```python
from build123d import *

# Parameters (mm, degrees)
F1_DEPTH     = 15
F3_DEPTH     = 6
F5_DEPTH     = 18
F6_R         = 10
F9_DEPTH     = 6
F10_DEPTH    = 6
F11_R        = 2
F13_DEPTH    = 6
F15_R        = 10
F19_DEPTH    = 45.001
F21_DEPTH    = 40.001
F23_DEPTH    = 6
F24_T1_DEPTH = 6


# Not quite as in the source:
# - a fillet or chamfer that OpenCascade refuses, or shapes differently, is made with other operations: its cross-section is extruded or revolved along the edge and cut away or added


with BuildPart() as f1:
    # F0 (on Front) → F1 (new body, symmetric)
    with BuildSketch(Plane.XZ):
        Polygon((9, -15), (9, 15), (3, 15), (3, 25), (-3, 25), (-3, 15), (-9, 15), (-9, -15), (-9, -25), (-3, -25), (-3, -15), (3, -15), (3, -25), (9, -25), align=None)
    extrude(amount=F1_DEPTH, both=True)

    # F2 (on face) → F3 (cut)
    with BuildSketch(Plane(origin=(-3, 0, 0), x_dir=(0, -1, 0), z_dir=(-1, 0, 0))):
        with BuildLine():
            ThreePointArc((0, 22.62), (-2.62, 20), (0, 17.38))
            Line((0, 17.38), (0, 22.62))
        make_face()
        with BuildLine():
            Line((0, 22.62), (0, 17.38))
            ThreePointArc((0, 17.38), (1.8526197667, 18.1473802333), (2.62, 20))
            ThreePointArc((2.62, 20), (1.8526197667, 21.8526197667), (0, 22.62))
        make_face()
    extrude(amount=-F3_DEPTH, mode=Mode.SUBTRACT)

    # F4 (on face) → F5 (cut)
    with BuildSketch(Plane(origin=(-9, 0, 0), x_dir=(0, -1, 0), z_dir=(-1, 0, 0))):
        with BuildLine():
            ThreePointArc((0, -22.62), (1.8526197667, -21.8526197667), (2.62, -20))
            ThreePointArc((2.62, -20), (-1.8526197667, -18.1473802333), (0, -22.62))
        make_face()
    extrude(amount=-F5_DEPTH, mode=Mode.SUBTRACT)

    # F6
    f6_edges = [f1.edges().sort_by_distance(p)[0] for p in [
        (0, 15, 25),
        (0, -15, 25),
        (6, -15, -25),
        (-6, -15, -25),
    ]]
    fillet(f6_edges, radius=F6_R)

    # F8 (on face) → F9 (cut)
    with BuildSketch(Plane(origin=(-9, 0, 0), x_dir=(0, -1, 0), z_dir=(-1, 0, 0))):
        with BuildLine():
            ThreePointArc((-7, 13.5872004348), (-5.1915204429, 7.8514360713), (-0.4202014333, 4.190274227))
            Line((-0.4202014333, 4.190274227), (15, -1.4222201011))
            Line((15, -1.4222201011), (15, 15))
            Line((15, 15), (-7, 15))
            Line((-7, 15), (-7, 13.5872004348))
        make_face()
    extrude(amount=-F9_DEPTH, mode=Mode.SUBTRACT)

    # F7 (on face) → F10 (cut)
    with BuildSketch(Plane.YZ.offset(9)):
        with BuildLine():
            Line((7, 15), (-15, 15))
            Line((-15, 15), (-15, -1.42222))
            Line((-15, -1.42222), (0.4202014333, 4.1902743281))
            ThreePointArc((0.4202014333, 4.1902743281), (5.1915204429, 7.8514361724), (7, 13.587200536))
            Line((7, 13.587200536), (7, 15))
        make_face()
    extrude(amount=-F10_DEPTH, mode=Mode.SUBTRACT)

    # F11
    f11_edges = [f1.edges().sort_by_distance(p)[0] for p in [
        (9, 15, -5),
        (-9, 15, -5),
    ]]
    fillet(f11_edges, radius=F11_R)

    # F12 (on face) → F13 (cut)
    with BuildSketch(Plane(origin=(-3, 0, 0), x_dir=(0, -1, 0), z_dir=(-1, 0, 0))):
        with BuildLine():
            Line((5, 25), (0, 25))
            ThreePointArc((0, 25), (3.5355339059, 23.5355339059), (5, 20))
            Line((5, 20), (5, 2.2174822415))
            Line((5, 2.2174822415), (15, -1.4222201011))
            Line((15, -1.4222201011), (15, 15))
            ThreePointArc((15, 15), (12.0710678119, 22.0710678119), (5, 25))
        make_face()
    extrude(amount=-F13_DEPTH, mode=Mode.SUBTRACT)

    # F15
    f15_edges = [f1.edges().sort_by_distance(p)[0] for p in [
        (0, -15, -15),
    ]]
    fillet(f15_edges, radius=F15_R)

    # F18 (on face) → F19 (cut, through all)
    with BuildSketch(Plane.XY.offset(20)):
        with BuildLine():
            ThreePointArc((2, -10), (1.4142135624, -8.5857864376), (0, -8))
            Line((0, -8), (0, -12))
            ThreePointArc((0, -12), (1.4142135624, -11.4142135624), (2, -10))
        make_face()
        with BuildLine():
            Line((0, -12), (0, -8))
            ThreePointArc((0, -8), (-2, -10), (0, -12))
        make_face()
    extrude(amount=-F19_DEPTH, mode=Mode.SUBTRACT)

    # F20 (on face) → F21 (cut, through all)
    with BuildSketch(Plane(origin=(0, 0, -15), x_dir=(1, 0, 0), z_dir=(0, 0, -1))):
        with BuildLine():
            ThreePointArc((0, -9), (-2, -11), (0, -13))
            Line((0, -13), (0, -11))
            Line((0, -11), (0, -9))
        make_face()
        with BuildLine():
            Line((0, -11), (0, -13))
            ThreePointArc((0, -13), (1.4142135624, -12.4142135624), (2, -11))
            ThreePointArc((2, -11), (1.4142135624, -9.5857864376), (0, -9))
            Line((0, -9), (0, -11))
        make_face()
    extrude(amount=-F21_DEPTH, mode=Mode.SUBTRACT)

    # F22 (on face) → F23 (cut)
    with BuildSketch(Plane.YZ.offset(3)):
        with BuildLine():
            ThreePointArc((0, 15), (-3.5355339059, 16.4644660941), (-5, 20))
            Line((-5, 20), (-5, 2.2174822415))
            Line((-5.0000000325, 2.2174823308), (0, 4.037333514))
            Line((0, 4.037333514), (0, 15))
        make_face()
    extrude(amount=-F23_DEPTH, mode=Mode.SUBTRACT)

    # F24: fillet of radius 5 on 2 edges, made by hand

    # F24_s2 → F24_t1 (join)
    with BuildSketch(Plane.YZ.offset(-3)):
        with BuildLine():
            ThreePointArc((-2.5, 15.6698729811), (-0.6698729811, 13.8397459622), (0, 11.3397459622))
            Line((0, 11.3397459622), (0, 15))
            ThreePointArc((0, 15), (-1.2940952255, 15.1703708686), (-2.5, 15.6698729811))
        make_face()
        with BuildLine():
            ThreePointArc((-3.2898992834, 2.8399081011), (-0.9042397786, 4.6704890233), (0, 7.538371205))
            Line((0, 7.538371205), (0, 4.037333514))
            Line((0, 4.037333514), (-3.2898992834, 2.8399081011))
        make_face()
    extrude(amount=F24_T1_DEPTH)


solid = f1.part
```
CAD build for the part. Positions are in the model's coordinates, mm. A direction names the side the tool comes from. Round coordinates to 2 decimals unless told otherwise and drop trailing zeros. Loops run counter-clockwise (first coordinate to the right, second up) from the corner with the lowest first, then second, coordinate; pieces in that order, holes last. Notation, with made-up numbers: M -5.75,-15 L 32.25,-15 A19 ccw 32.25,-5 Z; hole C 73,28.25 d1. An arc over 180 degrees is marked long. Use a Markdown table: item, result. Add a question column.
(1) Which spindle directions (+Z, -Z, +X, -X, +Y, -Y) get a long thin tool onto all of the face, cutting with end or side? Do faces 1 (the face through (0, 0, 9)), 2 (the face through (6, 7, 14)), 3 (the face through (6, 11, 15)), 4 (the face through (0, 5, -15)). Say none if no direction does.
(2) Pull direction X, two halves, no side cores. Call faces 5 (the face through (8.4, 14.43, -4.72)), 6 (the face through (0, -13, -11)), 7 (the face through (-8.4, 14.43, -5.28)): +X half, -X half, draft (parallel to the pull), parting line (faces both ways), or undercut.
(3) Drill centre lines: line 1 (Y direction, x = -4.2, z = -20); line 2 (X direction, y = 10, z = -17); line 3 (Z direction, x = 5.25, y = -1.5). Where is each one in solid material? Low to high.
(4) Cut at A-A (x = 4). Give the cut face in (y, z).
(5) Cut at C-C (z = -10). Give the cut face in (x, y), and give its area (3 significant figures).
(6) Cut at D-D (x = -0.75). Give the cut face in (y, z).
(7) Cut at B-B (z = -18). Give the cut face in (x, y).
(8) Flat gauge pins, fed straight in: pin 1 (10 mm diameter, centred on y = 1.5, z = 12.5, fed in from -X); pin 2 (3 mm diameter, centred on x = -5, y = 9, fed in from +Z); pin 3 (1.8 mm diameter, centred on x = 1.5, y = 2, fed in from -Z). Where does each tip first touch, or does it go through?
Geometry says:
| question | item | result |
|---|---|---|
| 1 | face 1 | +X, -X, -Y |
| 1 | face 2 | +Z, +X, -Y |
| 1 | face 3 | +Z, +X, +Y, -Y |
| 1 | face 4 | -Z, +Y, -Y |
| 2 | face 5 | +X half |
| 2 | face 6 | undercut |
| 2 | face 7 | -X half |
| 3 | line 1 | y = -13.66 to -2.62, 2.62 to 15 |
| 3 | line 2 | x = -9 to -3, 3 to 9 |
| 3 | line 3 | z = -25 to -22.15, -17.85 to 3.49 |
| 4 | outline | M -15,-15 A10 ccw -5,-25 L 15,-25 L 15,15 L 7,15 L 7,13.59 A10 cw 0.42,4.19 L -15,-1.42 Z; hole C 0,-20 d5.24 |
| 5 | outline | M -9,-15 L -3,-15 L -3,-13.66 L 3,-13.66 L 3,-15 L 9,-15 L 9,13 A2 ccw 7,15 L -7,15 A2 ccw -9,13 Z; hole C 0,-10 d4; hole C 0,11 d4 |
| 5 | area | 505 mm² |
| 6 | outline | M -15,-5 A10 ccw -11.85,-12.28 L -11.85,-0.28 L -15,-1.42 Z; M -8.15,-14.49 A10 ccw -5,-15 L 9.15,-15 L 9.15,24.1 A10 ccw 5,25 L 0,25 A5 ccw -2.5,15.67 A5 cw 0,11.34 L 0,7.54 A5 cw -3.29,2.84 L -8.15,1.07 Z; M 12.85,-15 L 15,-15 L 15,15 A10 ccw 12.85,21.19 Z; hole C 0,20 d5.24 |
| 7 | outline | M -9,-14.54 L -3,-14.54 L -3,-1.69 L -9,-1.69 Z; M -9,1.69 L -3,1.69 L -3,15 L -7,15 A2 ccw -9,13 Z; M 3,-14.54 L 9,-14.54 L 9,-1.69 L 3,-1.69 Z; M 3,1.69 L 9,1.69 L 9,13 A2 ccw 7,15 L 3,15 Z |
| 8 | pin 1 | stops at x = -3 |
| 8 | pin 2 | stops at z = 15 |
| 8 | pin 3 | stops at z = -15 |
